Could you check a few things on this model? Use its own coordinates, in mm. Face numbers are marked on the shaded views. A direction names the side the tool comes from. Round coordinates to 2 decimals unless told otherwise and drop trailing zeros. Loops run counter-clockwise (first coordinate to the right, second up) from the corner with the lowest first, then second, coordinate; pieces in that order, holes last. Notation, with made-up numbers: (88, 6.5) - (143, 6.5) arc R15 ccw to (143, 16.5) - close; hole circle Ø2 at (12, 65). An arc over 180 degrees is marked (long way). Answer as CSV lines item,"result". Start each with the question number.
1) Please list where these lines run through material, in increasing order: line 1 along X through (y, z) = (3.5, 0); line 2 along X through (y, z) = (4, 2); line 3 along X through (y, z) = (0.6, 0.5).
2) I'm going to push flat-ended pins straight in: pin 1 Ø2 at (y, z) = (3, 1.5) entering from -X; pin 2 Ø2 at (x, y) = (-11.5, 3) entering from -Z; pin 3 Ø1.5 at (x, y) = (-3.5, 3) entering from -Z. Where does each tip first touch, or does it pass through?
3) Suppose I cut it at B-B, the plane y = 3.45. Write out the boundary of the cut face in (x, z), then the cut area to 3 significant figures.
4) Suppose I cut it at A-A, the plane z = 2.5. Write out the boundary of the cut face in (x, y).
5) Suppose I cut it at C-C, the plane x = -15. Write out the boundary of the cut face in (y, z), then the cut area to 3 significant figures.
6) Which directions (+Z, -Z, +X, -X, +Y, -Y) give clear straight access to the entire face, cutting with the end or side of a thin tool? Please do the marked faces 1, 2, 3 and 4.
7) We'd pull the mould along X, two halves only. Please class the marked faces 5, 6 and 7: pulls with the +X half, pulls with the -X half, needs draft (parallel to the pull), parting line crosses it, or undercut.
```python
from build123d import *

# Parameters (mm, degrees)
SKETCH1_R           = 1.25
BOSS_EXTRUDE1_DEPTH = 4.5


with BuildPart() as part:
    # Sketch1 → Boss-Extrude1 (new body)
    with BuildSketch(Plane(origin=(0, 0, 0), x_dir=(1, 0, 0), z_dir=(0, 1, 0))):
        with BuildLine():
            Line((2.4, 0), (2.4, -6.5))
            ThreePointArc((2.4, -6.5), (1.697056275, -8.197056275), (0, -8.9))
            Line((0, -8.9), (-20, -8.9))
            ThreePointArc((-20, -8.9), (-22.4, -6.5), (-20, -4.1))
            Line((-20, -4.1), (-11.8, -4.1))
            Line((-11.8, -4.1), (-11.8, 1.4))
            Line((-11.8, 1.4), (-9.8, 1.4))
            Line((-9.8, 1.4), (-6.8, 0.4))
            Line((-6.8, 0.4), (-6.8, 0.3))
            ThreePointArc((-6.8, 0.3), (-7.063603897, -0.336396103), (-7.7, -0.6))
            Line((-7.7, -0.6), (-7.8, -0.6))
            Line((-7.8, -0.6), (-7.8, -4.1))
            Line((-7.8, -4.1), (-2.4, -4.1))
            Line((-2.4, -4.1), (-2.4, 0))
            ThreePointArc((-2.4, 0), (0, 2.4), (2.4, 0))
        make_face()
        with Locations(Location((0, 0, 0), (0, 0, 270))):
            Circle(SKETCH1_R, mode=Mode.SUBTRACT)
    extrude(amount=BOSS_EXTRUDE1_DEPTH)


solid = part.part
```
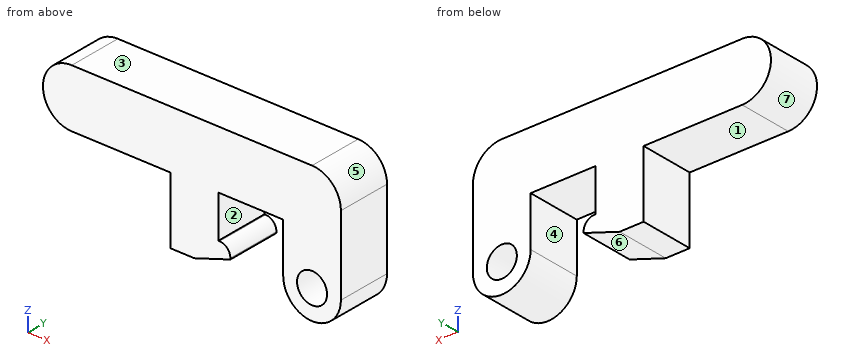
Filled sheet:
1,line 1,"-11.8 to -6.85, -2.4 to -1.25, 1.25 to 2.4"
1,line 2,"-11.8 to -7.8, -2.4 to 2.4"
1,line 3,"-11.8 to -7.29, -2.4 to -1.15, 1.15 to 2.4"
2,pin 1,"x = -11.8"
2,pin 2,"z = -1.4"
2,pin 3,"z = 4.1"
3,outline,"(-20, 4.1) - (-11.8, 4.1) - (-11.8, -1.4) - (-9.8, -1.4) - (-6.8, -0.4) - (-6.8, -0.3) arc R0.9 ccw to (-7.7, 0.6) - (-7.8, 0.6) - (-7.8, 4.1) - (-2.4, 4.1) - (-2.4, 0) arc R2.4 ccw to (2.4, 0) - (2.4, 6.5) arc R2.4 ccw to (0, 8.9) - (-20, 8.9) arc R2.4 ccw to start; hole circle Ø2.5 at (0, 0)"
3,area,"161 mm²"
4,outline,"(-11.8, 0) - (-7.8, 0) - (-7.8, 4.5) - (-11.8, 4.5) - close; (-2.4, 0) - (2.4, 0) - (2.4, 4.5) - (-2.4, 4.5) - close"
5,outline,"(0, 4.1) - (4.5, 4.1) - (4.5, 8.9) - (0, 8.9) - close"
5,area,"21.6 mm²"
6,face 1,"-Z, -X, +Y, -Y"
6,face 2,"+Y, -Y"
6,face 3,"+Z, +X, -X, +Y, -Y"
6,face 4,"-Z, +Y, -Y"
7,face 5,"pulls with the +X half"
7,face 6,"undercut"
7,face 7,"pulls with the -X half"
